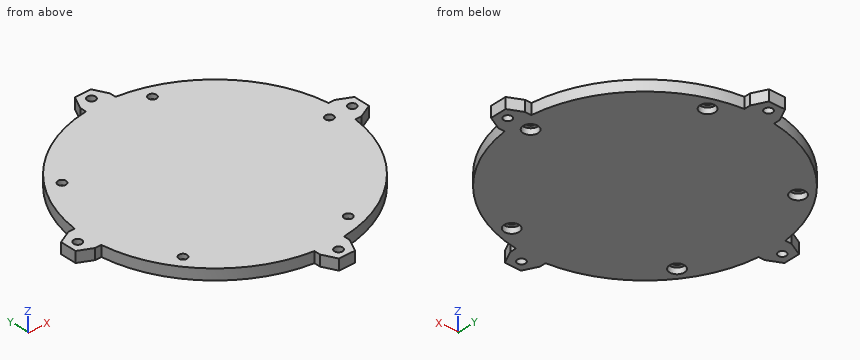
from build123d import *

# Parameters (mm, degrees)
SKETCH1_R           = 2.75
SKETCH1_R_2         = 1.5
BOSS_EXTRUDE2_DEPTH = 4
SKETCH1_4_R         = 2.75
SKETCH1_4_R_2       = 1.5
CUT_EXTRUDE1_DEPTH  = 2.2


with BuildPart() as part:
    # Sketch1 → Boss-Extrude2 (new body)
    with BuildSketch(Plane.XY):
        with BuildLine():
            Line((60, 5), (60, 7.319495552))
            ThreePointArc((60, 7.319495552), (88.087572106, 20.912427894), (101.680504448, 49))
            Line((101.680504448, 49), (104, 49))
            Line((104, 49), (109, 51.5))
            Line((109, 51.5), (109, 57.5))
            Line((109, 57.5), (104, 60))
            Line((104, 60), (101.680504448, 60))
            ThreePointArc((101.680504448, 60), (88.087572106, 88.087572106), (60, 101.680504448))
            Line((60, 101.680504448), (60, 104))
            Line((60, 104), (57.5, 109))
            Line((57.5, 109), (51.5, 109))
            Line((51.5, 109), (49, 104))
            Line((49, 104), (49, 101.680504448))
            ThreePointArc((49, 101.680504448), (20.912427894, 88.087572106), (7.319495552, 60))
            Line((7.319495552, 60), (5, 60))
            Line((5, 60), (0, 57.5))
            Line((0, 57.5), (0, 51.5))
            Line((0, 51.5), (5, 49))
            Line((5, 49), (7.319495552, 49))
            ThreePointArc((7.319495552, 49), (20.912427894, 20.912427894), (49, 7.319495552))
            Line((49, 7.319495552), (49, 5))
            Line((49, 5), (51.5, 0))
            Line((51.5, 0), (57.5, 0))
            Line((57.5, 0), (60, 5))
        make_face()
        with Locations((67.633222261, 14.080098057)):
            Circle(SKETCH1_R, mode=Mode.SUBTRACT)
        with Locations((97, 54.5)):
            Circle(SKETCH1_R, mode=Mode.SUBTRACT)
        with Locations((67.633222261, 94.919901943)):
            Circle(SKETCH1_R, mode=Mode.SUBTRACT)
        with Locations((20.116777739, 29.519126778)):
            Circle(SKETCH1_R, mode=Mode.SUBTRACT)
        with Locations((20.116777739, 79.480873222)):
            Circle(SKETCH1_R, mode=Mode.SUBTRACT)
        with Locations((54.5, 105.5)):
            Circle(SKETCH1_R_2, mode=Mode.SUBTRACT)
        with Locations((105.5, 54.5)):
            Circle(SKETCH1_R_2, mode=Mode.SUBTRACT)
        with Locations((3.5, 54.5)):
            Circle(SKETCH1_R_2, mode=Mode.SUBTRACT)
        with Locations((54.5, 3.5)):
            Circle(SKETCH1_R_2, mode=Mode.SUBTRACT)
        with Locations((20.116777739, 79.480873222)):
            Circle(SKETCH1_R)
        with Locations((20.116777739, 79.480873222)):
            Circle(SKETCH1_R_2, mode=Mode.SUBTRACT)
        with Locations((67.633222261, 94.919901943)):
            Circle(SKETCH1_R)
        with Locations((67.633222261, 94.919901943)):
            Circle(SKETCH1_R_2, mode=Mode.SUBTRACT)
        with Locations((97, 54.5)):
            Circle(SKETCH1_R)
        with Locations((97, 54.5)):
            Circle(SKETCH1_R_2, mode=Mode.SUBTRACT)
        with Locations((67.633222261, 14.080098057)):
            Circle(SKETCH1_R)
        with Locations((67.633222261, 14.080098057)):
            Circle(SKETCH1_R_2, mode=Mode.SUBTRACT)
        with Locations((20.116777739, 29.519126778)):
            Circle(SKETCH1_R)
        with Locations((20.116777739, 29.519126778)):
            Circle(SKETCH1_R_2, mode=Mode.SUBTRACT)
    extrude(amount=BOSS_EXTRUDE2_DEPTH)

    # Sketch1_4 → Cut-Extrude1 (cut)
    with BuildSketch(Plane.XY):
        with Locations((20.116777739, 29.519126778)):
            Circle(SKETCH1_4_R)
        with Locations((20.116777739, 29.519126778)):
            Circle(SKETCH1_4_R_2, mode=Mode.SUBTRACT)
        with Locations((67.633222261, 14.080098057)):
            Circle(SKETCH1_4_R)
        with Locations((67.633222261, 14.080098057)):
            Circle(SKETCH1_4_R_2, mode=Mode.SUBTRACT)
        with Locations((97, 54.5)):
            Circle(SKETCH1_4_R)
        with Locations((97, 54.5)):
            Circle(SKETCH1_4_R_2, mode=Mode.SUBTRACT)
        with Locations((67.633222261, 94.919901943)):
            Circle(SKETCH1_4_R)
        with Locations((67.633222261, 94.919901943)):
            Circle(SKETCH1_4_R_2, mode=Mode.SUBTRACT)
        with Locations((20.116777739, 79.480873222)):
            Circle(SKETCH1_4_R)
        with Locations((20.116777739, 79.480873222)):
            Circle(SKETCH1_4_R_2, mode=Mode.SUBTRACT)
    extrude(amount=CUT_EXTRUDE1_DEPTH, mode=Mode.SUBTRACT)


solid = part.part
The model under review builds one solid part; all positions refer to its coordinate system, in mm. Round coordinates to 2 decimals unless told otherwise and drop trailing zeros. Loops run counter-clockwise (first coordinate to the right, second up) from the corner with the lowest first, then second, coordinate; pieces in that order, holes last. Notation, with made-up numbers: (53, 31.5) -> (96, 31.5) arc R25 ccw to (96, 59.5) -> close; hole circle Ø7 at (-23.5, -13.75). An arc over 180 degrees is marked (long way). Write item = value, one per line. Start each with the question number.
Item 1: Take a section at D-D on x = 97. Give the boundary of the cut face in (y, z), plus the area to 3 significant figures.
Item 2: To check wall thickness, follow L1, parallel to Y at x = 54.5, z = 1.05; L2, parallel to Y at x = 68.5, z = 3.3; L3, parallel to X at y = 30.5, z = 2.65. State the ranges of each line that lie inside material, in increasing order.
Item 3: Take a section at A-A on y = 3.5. Give the boundary of the cut face in (x, z), plus the area to 3 significant figures.
Item 4: Insertion check: pin 1 (1.2 mm diameter, centred on x = 6, z = 1.5, fed in from -Y); pin 2 (0.7 mm diameter, centred on x = 6, z = 1.5, fed in from +Y); pin 3 (6 mm diameter, centred on x = 51, y = 45, fed in from -Z); pin 4 (1.9 mm diameter, centred on y = 6, z = 1.5, fed in from +X). Each pin has a flat end and moves straight along its axis. Give the tip position at first contact, or say it passes through.
Item 5: Take a section at C-C on z = 3.1. Count the separate pieces of the cut face and the enclosed holes in it, plus the area to 3 significant figures.
Result:
q1.outline = (33.29, 0) -> (51.75, 0) -> (51.75, 2.2) -> (53, 2.2) -> (53, 4) -> (33.29, 4) -> close; (56, 2.2) -> (57.25, 2.2) -> (57.25, 0) -> (75.71, 0) -> (75.71, 4) -> (56, 4) -> close
q1.area = 152 mm²
q2.L1 = 0 to 2, 5 to 104, 107 to 109
q2.L2 = 9.11 to 12.86, 15.3 to 93.7, 96.14 to 99.89
q2.L3 = 13.51 to 18.98, 21.25 to 95.49
q3.outline = (49.75, 0) -> (53, 0) -> (53, 4) -> (49.75, 4) -> close; (56, 0) -> (59.25, 0) -> (59.25, 4) -> (56, 4) -> close
q3.area = 26.0 mm²
q4.pin_1 = 49
q4.pin_2 = 60
q4.pin_3 = 0
q4.pin_4 = 60
q5.separate_pieces = 1
q5.enclosed_holes = 9
q5.area = 7,290 mm²
